```python
from build123d import *

# Parameters (mm, degrees)
SKETCH1_W           = 8.5
SKETCH1_H           = 12
BOSS_EXTRUDE1_DEPTH = 41.5
CUT_EXTRUDE1_DEPTH  = 43.784342931
FILLET1_R           = 0.5
M2_HOLE1_R_D        = 1.6
M2_HOLE1_R_DEPTH    = 5
M2_HOLE1_R_TIP      = 0.480688495
M2_HOLE2_T_D        = 1.6
M2_HOLE2_T_DEPTH    = 4
M2_HOLE2_T_TIP      = 0.480688495
M2_HOLE3_U_D        = 2.4
M2_HOLE3_U_DEPTH    = 10
M2_HOLE3_U_TIP      = 0.721032743
M2_HOLE4_V_D        = 1.6
M2_HOLE5_W_D        = 1.6
M2_HOLE5_W_DEPTH    = 5
M2_HOLE5_W_TIP      = 0.480688495
M2_HOLE6_Y_D        = 2.4
M2_HOLE6_Y_DEPTH    = 10
M2_HOLE6_Y_TIP      = 0.721032743


with BuildPart() as part:
    # Sketch1 → Boss-Extrude1 (new, symmetric)
    with BuildSketch(Plane.XY):
        Rectangle(SKETCH1_W, SKETCH1_H)
    extrude(amount=BOSS_EXTRUDE1_DEPTH, both=True)

    # Sketch2 → Cut-Extrude1 (cut, through all)
    with BuildSketch(Plane(origin=(4.25, 0, 0), x_dir=(0, 0, -1), z_dir=(1, 0, 0))):
        with BuildLine():
            Line((-37.5, 1), (37.5, 1))
            ThreePointArc((37.5, 1), (38.207106781, 0.707106781), (38.5, 0))
            Line((38.5, 0), (38.5, -6))
            Line((38.5, -6), (-38.5, -6))
            Line((-38.5, -6), (-38.5, 0))
            ThreePointArc((-38.5, 0), (-38.207106781, 0.707106781), (-37.5, 1))
        make_face()
    extrude(amount=-CUT_EXTRUDE1_DEPTH, mode=Mode.SUBTRACT)

    # Fillet1
    fillet1_edges = [part.edges().sort_by_distance(p)[0] for p in [
        (0, -6, 41.5),
        (0, -6, -38.5),
        (0, -6, 38.5),
        (0, -6, -41.5),
        (0, 6, -41.5),
        (0, 6, 41.5),
    ]]
    fillet(fillet1_edges, radius=FILLET1_R)

    # M2 Hole1-R
    with Locations(Plane(origin=(4.25, 0, 0), x_dir=(0, 0, -1), z_dir=(1, 0, 0))):
        with Locations((21.5, 3.5), (-21.5, 3.5)):
            Hole(M2_HOLE1_R_D / 2, depth=M2_HOLE1_R_DEPTH)
            with Locations((0, 0, -(M2_HOLE1_R_DEPTH + M2_HOLE1_R_TIP / 2))):  # 118° drill point
                Cone(0, M2_HOLE1_R_D / 2, M2_HOLE1_R_TIP, mode=Mode.SUBTRACT)

    # M2 Hole2-T
    with Locations(Plane(origin=(4.25, 0, 0), x_dir=(0, 0, -1), z_dir=(1, 0, 0))):
        with Locations((0, 3.5)):
            Hole(M2_HOLE2_T_D / 2, depth=M2_HOLE2_T_DEPTH)
            with Locations((0, 0, -(M2_HOLE2_T_DEPTH + M2_HOLE2_T_TIP / 2))):  # 118° drill point
                Cone(0, M2_HOLE2_T_D / 2, M2_HOLE2_T_TIP, mode=Mode.SUBTRACT)

    # M2 Hole3-U
    with Locations(Plane.XY.offset(41.5)):
        with Locations((0, -3)):
            Hole(M2_HOLE3_U_D / 2, depth=M2_HOLE3_U_DEPTH)
            with Locations((0, 0, -(M2_HOLE3_U_DEPTH + M2_HOLE3_U_TIP / 2))):  # 118° drill point
                Cone(0, M2_HOLE3_U_D / 2, M2_HOLE3_U_TIP, mode=Mode.SUBTRACT)

    # M2 Hole4-V (through all)
    with Locations(Plane(origin=(0, 6, 0), x_dir=(1, 0, 0), z_dir=(0, 1, 0))):
        with Locations((0, 29), (0, -29)):
            Hole(M2_HOLE4_V_D / 2)

    # M2 Hole5-W
    with Locations(Plane.ZY.offset(4.25)):
        with Locations((-35.5, 3.5), (35.5, 3.5)):
            Hole(M2_HOLE5_W_D / 2, depth=M2_HOLE5_W_DEPTH)
            with Locations((0, 0, -(M2_HOLE5_W_DEPTH + M2_HOLE5_W_TIP / 2))):  # 118° drill point
                Cone(0, M2_HOLE5_W_D / 2, M2_HOLE5_W_TIP, mode=Mode.SUBTRACT)

    # M2 Hole6-Y
    with Locations(Plane(origin=(0, 0, -41.5), x_dir=(-1, 0, 0), z_dir=(0, 0, -1))):
        with Locations((0, -3)):
            Hole(M2_HOLE6_Y_D / 2, depth=M2_HOLE6_Y_DEPTH)
            with Locations((0, 0, -(M2_HOLE6_Y_DEPTH + M2_HOLE6_Y_TIP / 2))):  # 118° drill point
                Cone(0, M2_HOLE6_Y_D / 2, M2_HOLE6_Y_TIP, mode=Mode.SUBTRACT)


solid = part.part
```
Work out the finished part from the listing and answer in its coordinate system (mm). A direction names the side the tool comes from. Round coordinates to 2 decimals unless told otherwise and drop trailing zeros. Order: outer loops, then holes, each group sorted by start corner. A loop starts at its lowest first (then second) coordinate and runs counter-clockwise, first axis right, second up.
Q1. A cutting plane is placed at A-A, the plane z = -29. Determine the outline of the cut face in (x, y), then the cut area to 3 significant figures.
Solution:
outline: (-4.25, 1) - (-0.8, 1) - (-0.8, 6) - (-4.25, 6) - close; (0.8, 1) - (4.25, 1) - (4.25, 6) - (0.8, 6) - close
area: 34.5 mm2
Q2. Given pin 1 Ø1.9 at (x, y) = (0, -3) entering from +Z; pin 2 Ø1.8 at (y, z) = (3.5, 21.5) entering from +X; pin 3 Ø1.3 at (y, z) = (3.5, 0) entering from +X; pin 4 Ø2.5 at (x, z) = (0, -29) entering from -Y, each flat-ended and moving along its own axis, determine where each tip first touches the part or whether it passes through.
Solution:
pin 1: passes through
pin 2: stops at x = 4.25
pin 3: stops at x = 0.16
pin 4: stops at y = 1
Q3. A cutting plane is placed at D-D, the plane z = -2. Determine the outline of the cut face in (x, y), then the cut area to 3 significant figures.
Solution:
outline: (-4.25, 1) - (4.25, 1) - (4.25, 6) - (-4.25, 6) - close
area: 42.5 mm2
Q4. Find the intervals of material crossed by line 1 along Z through (x, y) = (3.25, 3.5); line 2 along Z through (x, y) = (1.25, -1); line 3 along Z through (x, y) = (-4, 3.75), in increasing order.
Solution:
line 1: z = -41.5 to -22.3, -20.7 to -0.8, 0.8 to 20.7, 22.3 to 41.5
line 2: z = -41.5 to -38.5, 38.5 to 41.5
line 3: z = -41.5 to -36.26, -34.74 to 34.74, 36.26 to 41.5
Q5. A cutting plane is placed at C-C, the plane x = 2.25. Determine the outline of the cut face in (y, z), then the cut area to 3 significant figures.
Solution:
outline: (-6, -41) arc R0.5 ccw to (-5.5, -41.5) - (5.5, -41.5) arc R0.5 ccw to (6, -41) - (6, 41) arc R0.5 ccw to (5.5, 41.5) - (-5.5, 41.5) arc R0.5 ccw to (-6, 41) - (-6, 39) arc R0.5 ccw to (-5.5, 38.5) - (0, 38.5) arc R1 cw to (1, 37.5) - (1, -37.5) arc R1 cw to (0, -38.5) - (-5.5, -38.5) arc R0.5 ccw to (-6, -39) - close; hole circle Ø1.6 at (3.5, -21.5); hole circle Ø1.6 at (3.5, 0); hole circle Ø1.6 at (3.5, 21.5)
area: 451 mm2
Q6. The mould has two halves that part along Y. Classify faces 5 (the cylindrical face through (0.16, -1.81, 39.98)), 6 (the flat face through (0, -6, -40)), 7 (the flat face through (4.25, 3, 1)): pulls with the +Y half, pulls with the -Y half, needs draft (parallel to the pull), parting line crosses it, or undercut.
Solution:
face 5: undercut
face 6: pulls with the -Y half
face 7: needs draft
Q7. A tool of negligible diameter and unlimited length cuts with its end or side. For faces 1 (the cylindrical face through (1.72, 2.72, -21.67)), 2 (the cylindrical face through (-1.715, 3.74, 34.737)), 3 (the flat face through (1, -2, 38.5)), 4 (the flat face through (0, 0, 41.5)), from which of +Z, -Z, +X, -X, +Y, -Y can it reach the whole face along a straight path? Write none if from no direction.
Solution:
face 1: +X
face 2: -X
face 3: +X, -X, -Y
face 4: +Z, +X, -X, +Y, -Y
Q8. A cutting plane is placed at B-B, the plane x = -2.5. Determine the outline of the cut face in (y, z).
Solution:
outline: (-6, -41) arc R0.5 ccw to (-5.5, -41.5) - (5.5, -41.5) arc R0.5 ccw to (6, -41) - (6, 41) arc R0.5 ccw to (5.5, 41.5) - (-5.5, 41.5) arc R0.5 ccw to (-6, 41) - (-6, 39) arc R0.5 ccw to (-5.5, 38.5) - (0, 38.5) arc R1 cw to (1, 37.5) - (1, -37.5) arc R1 cw to (0, -38.5) - (-5.5, -38.5) arc R0.5 ccw to (-6, -39) - close; hole circle Ø1.6 at (3.5, -35.5); hole circle Ø1.6 at (3.5, 35.5)
